Could you check a few things on this model? Use its own coordinates, in mm. A direction names the side the tool comes from. Coordinates: 2 decimals unless noted, no trailing zeros. Order: outer loops, then holes, each group sorted by start corner. A loop starts at its lowest first (then second) coordinate and runs counter-clockwise, first axis right, second up. Notation, with made-up numbers: (73.25, 64.25) -> (78.25, 64.25) arc R14 ccw to (78.25, 86.25) -> close; hole circle Ø8 at (-38.5, 60). An arc over 180 degrees is marked (long way). Return JSON: item names as keys, results as strings. Group by question number.
from build123d import *

# Parameters (mm, degrees)
F1_DEPTH = 9
F2_W     = 7
F2_H     = 1.55604
F3_DEPTH = 2
F5_DEPTH = 9
F6_DEPTH = 9
F8_DEPTH = 2


with BuildPart() as f1:
    # F0 (on Front) → F1 (new body)
    with BuildSketch(Plane.XZ):
        with BuildLine():
            Line((17, -7.35), (17, 7.35))
            ThreePointArc((17, 7.35), (15.755204, 10.355204), (12.75, 11.6))
            Line((12.75, 11.6), (-12.75, 11.6))
            ThreePointArc((-12.75, 11.6), (-15.755204, 10.355204), (-17, 7.35))
            Line((-17, 7.35), (-17, -7.35))
            ThreePointArc((-17, -7.35), (-15.755204, -10.355204), (-12.75, -11.6))
            Line((-12.75, -11.6), (12.75, -11.6))
            ThreePointArc((12.75, -11.6), (15.755204, -10.355204), (17, -7.35))
        make_face()
        with BuildLine():
            ThreePointArc((16, -7.35), (15.048097, -9.648097), (12.75, -10.6))
            Line((12.75, -10.6), (-12.75, -10.6))
            ThreePointArc((-12.75, -10.6), (-15.048097, -9.648097), (-16, -7.35))
            Line((-16, -7.35), (-16, 7.35))
            ThreePointArc((-16, 7.35), (-15.048097, 9.648097), (-12.75, 10.6))
            Line((-12.75, 10.6), (12.75, 10.6))
            ThreePointArc((12.75, 10.6), (15.048097, 9.648097), (16, 7.35))
            Line((16, 7.35), (16, -7.35))
        make_face(mode=Mode.SUBTRACT)
    extrude(amount=F1_DEPTH)

    # F2 (on face) → F3 (join)
    with BuildSketch(Plane.XY.offset(11.6)):
        with Locations((0, -8.22198)):
            Rectangle(F2_W, F2_H)
    extrude(amount=F3_DEPTH)

    # F4 (on Front) → F5 (join)
    with BuildSketch(Plane.XZ):
        with BuildLine():
            Line((-11.904627, 10.6), (-12.75, 10.6))
            ThreePointArc((-12.75, 10.6), (-12.327314, 10.469545), (-11.904627, 10.6))
        make_face()
        with BuildLine():
            ThreePointArc((11.904627, 10.6), (12.327314, 10.469545), (12.75, 10.6))
            Line((12.75, 10.6), (11.904627, 10.6))
        make_face()
    extrude(amount=F5_DEPTH)

    # F4 (on Front) → F6 (join)
    with BuildSketch(Plane.XZ):
        with BuildLine():
            Line((-11.904627, 10.6), (-12.75, 10.6))
            ThreePointArc((-12.75, 10.6), (-12.327314, 10.469545), (-11.904627, 10.6))
        make_face()
        with BuildLine():
            ThreePointArc((11.904627, 10.6), (12.327314, 10.469545), (12.75, 10.6))
            Line((12.75, 10.6), (11.904627, 10.6))
        make_face()
    extrude(amount=F6_DEPTH)

    # F7 (on face) → F8 (join)
    with BuildSketch(Plane(origin=(0, 0, -11.6), x_dir=(1, 0, 0), z_dir=(0, 0, -1))):
        Polygon((3.5, 9), (0, 9), (-3.5, 9), (-3.5, 7.44), (0, 7.44), (3.5, 7.44), align=None)
    extrude(amount=F8_DEPTH)


solid = f1.part
Q1. On a 3-axis mill with a long thin cutter (end or side, diameter ignored), from which of +Z, -Z, +X, -X, +Y, -Y can I reach the whole of each face in a straight line? I mean faces 4 (the flat face through (3.5, -8, 13)), 5 (the cylindrical face through (-15.023, -4.437, -9.673)), 6 (the flat face through (0, -7.44, -13)), 7 (the flat face through (-3.5, -8, 13)), 8 (the flat face through (-3.5, -8, -13)). Say none if no direction works.
Q2. I want a section at B-B on z = 5. Please give me the cut outline in (x, y).
Q3. I want a section at C-C on y = -8. Please give me the cut outline in (x, z), and give its area (3 significant figures).
Q4. I want a section at A-A on x = 4.5. Please give me the cut outline in (y, z).
Q5. We'd pull the mould along Z, two halves only. Please class faces 1 (the cylindrical face through (-15.72, -4.44, 10.39)), 2 (the flat face through (0, -9, 11)), 3 (the cylindrical face through (12.32, -4.44, 10.47)): pulls with the +Z half, pulls with the -Z half, needs draft (parallel to the pull), parting line crosses it, or undercut.
Q6. I need wall thicknesses on line 1 along X through (y, z) = (-0.75, 1.75); line 2 along Z through (x, y) = (2.5, -1.25); line 3 along X through (y, z) = (-6.5, -9.75). Which ranges of each line are inside material? Lowest first, please. Write a range as from..to.
Q7. I want a section at D-D on z = 12.25. Please give me the cut outline in (x, y), and give its area (3 significant figures).
Q8. I'm going to push flat-ended pins straight in: pin 1 Ø0.5 at (y, z) = (-8, -12.5) entering from +X; pin 2 Ø2.5 at (x, y) = (0, -4.5) entering from -Z; pin 3 Ø3 at (y, z) = (-6.5, 9) entering from -X. Where does each tip first touch, or does it pass through?
Response values:
{
 "1": {"face 4": "+Z, +X, +Y, -Y", "face 5": "+Y, -Y", "face 6": "-Z, +X, -X, +Y", "face 7": "+Z, -X, +Y, -Y", "face 8": "-Z, -X, +Y, -Y"},
 "2": {"outline": "(-17, -9) -> (-16, -9) -> (-16, 0) -> (-17, 0) -> close; (16, -9) -> (17, -9) -> (17, 0) -> (16, 0) -> close"},
 "3": {"outline": "(-17, -7.35) arc R4.25 ccw to (-12.75, -11.6) -> (-3.5, -11.6) -> (-3.5, -13.6) -> (3.5, -13.6) -> (3.5, -11.6) -> (12.75, -11.6) arc R4.25 ccw to (17, -7.35) -> (17, 7.35) arc R4.25 ccw to (12.75, 11.6) -> (3.5, 11.6) -> (3.5, 13.6) -> (-3.5, 13.6) -> (-3.5, 11.6) -> (-12.75, 11.6) arc R4.25 ccw to (-17, 7.35) -> close; hole (-16, -7.35) arc R3.25 ccw to (-12.75, -10.6) -> (12.75, -10.6) arc R3.25 ccw to (16, -7.35) -> (16, 7.35) arc R3.25 ccw to (12.75, 10.6) arc R0.75 cw to (11.9, 10.6) -> (-11.9, 10.6) arc R0.75 cw to (-12.75, 10.6) arc R3.25 ccw to (-16, 7.35) -> close", "area": "132 mm²"},
 "4": {"outline": "(-9, -11.6) -> (0, -11.6) -> (0, -10.6) -> (-9, -10.6) -> close; (-9, 10.6) -> (0, 10.6) -> (0, 11.6) -> (-9, 11.6) -> close"},
 "5": {"face 1": "pulls with the +Z half", "face 2": "needs draft", "face 3": "undercut"},
 "6": {"line 1": "x = -17..-16, 16..17", "line 2": "z = -11.6..-10.6, 10.6..11.6", "line 3": "x = -16.26..-14.94, 14.94..16.26"},
 "7": {"outline": "(-3.5, -9) -> (3.5, -9) -> (3.5, -7.44) -> (-3.5, -7.44) -> close", "area": "10.9 mm²"},
 "8": {"pin 1": "stops at x = 3.5", "pin 2": "stops at z = -11.6", "pin 3": "stops at x = -17"}
}
